Print and shaded views of the part. All mm, measured from the part's lowest x, y and z. Round coordinates to 2 decimals unless told otherwise and drop trailing zeros. Order: outer loops, then holes, each group sorted by start corner. A loop starts at its lowest first (then second) coordinate and runs counter-clockwise, first axis right, second up. Notation, with made-up numbers: (7.5, -5) - (59.5, -5) arc R11 cw to (59.5, 5) - close; hole circle Ø9 at (54, 62.25). An arc over 180 degrees is marked (long way). Return JSON: item names as keys, results as strings. Group by question number.
Item 1: Saw through at B-B on y = 10. List the corners of the cut face in (x, z), and give its area (3 significant figures).
Item 2: Saw through at A-A on z = 7.5. List the corners of the cut face in (x, y), and give its area (3 significant figures).
Item 3: Probe probe 1 along X at (y, z) = (15, 18) (1 decimal); probe 2 along X at (y, z) = (21, 10) (1 decimal). List the from-to ranges inside material, lowest first.
Item 4: Drop flat-ended pins along their axis: pin 1 (2 mm diameter, centred on y = 19, z = 16, fed in from -X); pin 2 (3 mm diameter, centred on y = 12.5, z = 26, fed in from -X); pin 3 (6 mm diameter, centred on y = 14, z = 9.5, fed in from +X) (1 decimal). Give the stop position or say it passes through.
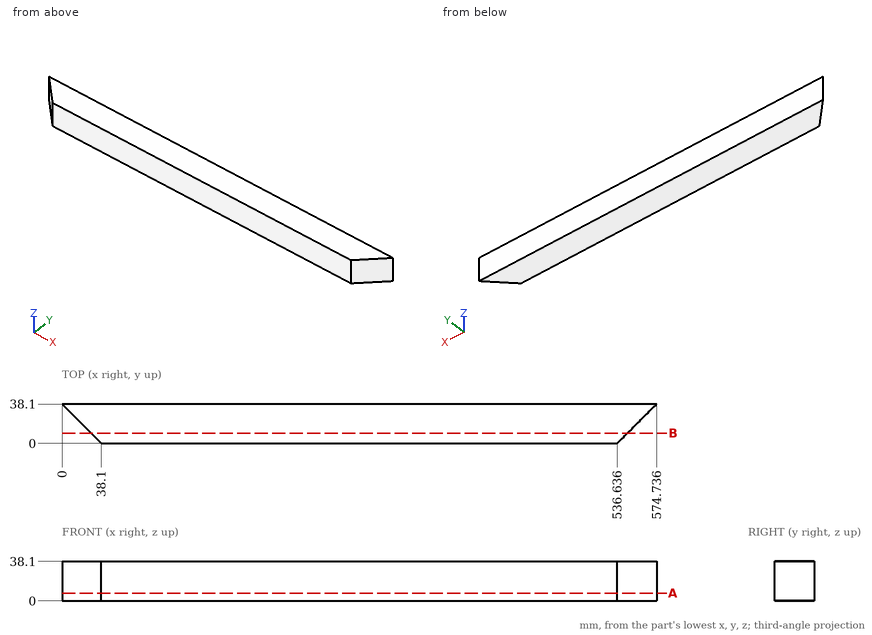
Filled in:
{
 "1": {"outline": "(28.1, 0) - (546.64, 0) - (546.64, 38.1) - (28.1, 38.1) - close", "area": "19,800 mm^2"},
 "2": {"outline": "(0, 38.1) - (38.1, 0) - (536.64, 0) - (574.74, 38.1) - close", "area": "20,400 mm^2"},
 "3": {"probe 1": "x = 23.1 to 551.6", "probe 2": "x = 17.1 to 557.6"},
 "4": {"pin 1": "stops at x = 18.1", "pin 2": "stops at x = 24.1", "pin 3": "stops at x = 553.6"}
}
